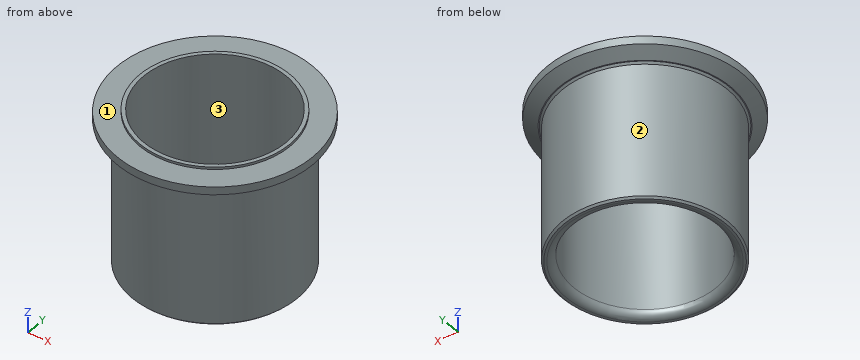
```python
from build123d import *

# Parameters (mm, degrees)
SKETCH2_R          = 30.175
CUT_EXTRUDE1_DEPTH = 88.694170274
CHAMFER1_SIZE      = 0.75
CHAMFER2_SIZE      = 3
CHAMFER2_SIZE2     = 5.196152423
FILLET1_R          = 3


with BuildPart() as part:
    # Sketch1 → Revolve1 (revolve)
    with BuildSketch(Plane(origin=(0, 0, 0), x_dir=(1, 0, 0), z_dir=(0, 1, 0)), mode=Mode.PRIVATE) as revolve1_sk:
        Polygon((0, 0), (0, 65.35), (-35, 65.35), (-35, 7.35), (-41.35, 7.35), (-41.35, 1), (-31.75, 1), (-31.75, 0), align=None)
    revolve(revolve1_sk.sketch.rotate(Axis((0, 0, 0), (0, 0, -1)), 180), axis=Axis((0, 0, 0), (0, 0, -1)))

    # Sketch2 → Cut-Extrude1 (cut, through all)
    with BuildSketch(Plane(origin=(0, 0, -65.35), x_dir=(-1, 0, 0), z_dir=(0, 0, -1))):
        Circle(SKETCH2_R)
    extrude(amount=-CUT_EXTRUDE1_DEPTH, mode=Mode.SUBTRACT)

    # Chamfer1
    chamfer1_edges = [part.edges().sort_by_distance(p)[0] for p in [
        (-35, 0, -7.35),
        (-35, 0, -65.35),
    ]]
    chamfer(chamfer1_edges, length=CHAMFER1_SIZE)

    # Chamfer2
    chamfer2_edges = [part.edges().sort_by_distance(p)[0] for p in [
        (-41.35, 0, -7.35),
    ]]
    chamfer2_side = [part.faces().sort_by_distance(p)[0] for p in [
        (-41.35, 0, -4.175),
    ]]
    chamfer(chamfer2_edges, length=CHAMFER2_SIZE, length2=CHAMFER2_SIZE2, reference=chamfer2_side[0])

    # Fillet1
    fillet1_edges = [part.edges().sort_by_distance(p)[0] for p in [
        (30.175, 0, -65.35),
    ]]
    fillet(fillet1_edges, radius=FILLET1_R)


solid = part.part
```
Check sheet for the modelled part. Datum: model origin and axes. Units: mm. Face numbers are marked on the shaded views. Coordinates: 2 decimals unless noted, no trailing zeros. Write each loop counter-clockwise with the first axis right and the second up, starting at its lowest first coordinate (ties: lowest second). Pieces come first, ordered by that corner, then holes. Notation, with made-up numbers: (-31, 43.5) -> (26, 43.5) arc R19 cw to (26, 64.5) -> close; hole circle Ø2 at (31.5, 21.5). An arc over 180 degrees is marked (long way). Use a Markdown table: item, result.
1. Sectioned sample at A-A (y = 0). Enter the section's corners in (x, z) (3 decimals), plus the area to 3 significant figures.
Reported:
| item | result |
|---|---|
| outline | (-41.35, -4.35) -> (-36.154, -7.35) -> (-35.75, -7.35) -> (-35, -8.1) -> (-35, -64.6) -> (-34.25, -65.35) -> (-33.175, -65.35) arc R3 ccw to (-30.175, -62.35) -> (-30.175, 0) -> (-31.75, 0) -> (-31.75, -1) -> (-41.35, -1) -> close; (30.175, -62.35) arc R3 ccw to (33.175, -65.35) -> (34.25, -65.35) -> (35, -64.6) -> (35, -8.1) -> (35.75, -7.35) -> (36.154, -7.35) -> (41.35, -4.35) -> (41.35, -1) -> (31.75, -1) -> (31.75, 0) -> (30.175, 0) -> close |
| area | 685 mm2 |
2. Go/stop test with flat-tipped pins: pin 1 Ø5 at (y, z) = (-17.5, -13) entering from +X; pin 2 Ø10 at (y, z) = (-27, -42.5) entering from +X; pin 3 Ø6 at (y, z) = (10, -35) entering from -X; pin 4 Ø12 at (x, y) = (-20, -24.5) entering from -Z. Record where each tip stops, or that it passes through.
Reported:
| item | result |
|---|---|
| pin 1 | stops at x = 31.62 |
| pin 2 | stops at x = 27.22 |
| pin 3 | stops at x = -34.29 |
| pin 4 | stops at z = -65.35 |
3. Release check for a two-part mould opening along Y. For the marked faces 1, 2 and 3 record: pulls with the +Y half, pulls with the -Y half, needs draft (parallel to the pull), parting line crosses it, or undercut.
Reported:
| item | result |
|---|---|
| face 1 | needs draft |
| face 2 | parting line crosses it |
| face 3 | undercut |
4. Sectioned sample at C-C (z = -28). Enter the section's corners in (x, y) (3 decimals).
Reported:
| item | result |
|---|---|
| outline | circle Ø70 at (0, 0); hole circle Ø60.35 at (0, 0) |
5. Scan lines: line 1 along Y through (x, z) = (0, -26.5) (3 decimals); line 2 along Z through (x, y) = (23, 23.5); line 3 along Y through (x, z) = (-15, -54.5). Record each from-to range of solid material in increasing order.
Reported:
| item | result |
|---|---|
| line 1 | y = -35 to -30.175, 30.175 to 35 |
| line 2 | z = -65.34 to -1 |
| line 3 | y = -31.62 to -26.18, 26.18 to 31.62 |
